Check sheet for the modelled part. Datum: model origin and axes. Units: mm. A direction names the side the tool comes from. Give positions to 0.01 mm unless a question says otherwise; leave off trailing zeros. Order: outer loops, then holes, each group sorted by start corner. A loop starts at its lowest first (then second) coordinate and runs counter-clockwise, first axis right, second up. Notation, with made-up numbers: (-20, -16) -> (13, -16) arc R29 cw to (13, 23) -> close; hole circle Ø3 at (84, -4.5). An arc over 180 degrees is marked (long way). Answer in a Markdown table with one row per item. Add a question column.
(1) Thickness scan on L1, parallel to X at y = 35, z = -40; L2, parallel to Z at x = 26, y = -19.5; L3, parallel to Y at x = -44, z = -14.5. Record the ranges inside material, lowest first. Write a range as [from, to].
(2) Cross-section at C-C (x = 0). Record the cut outline in (y, z).
(3) Go/stop test with flat-tipped pins: pin 1 (5 mm diameter, centred on x = 27.5, y = -14, fed in from -Z); pin 2 (5 mm diameter, centred on y = 11.5, z = 39.5, fed in from +X); pin 3 (1.5 mm diameter, centred on x = 36.5, z = -14, fed in from -Y). Record where each tip stops, or that it passes through.
(4) Release check for a two-part mould opening along Z. For faces 1 (the face through (-60.189, 2.649, 35.827)), 2 (the face through (60.189, 2.717, 35.827)), 3 (the face through (1.08, -4.88, -59.93)), 4 (the face through (0, 0, -65)) record: released by +Z, released by -Z, zero draft, split by the parting line, or undercut.
(5) Cross-section at B-B (y = -3). Record the cut outline in (x, z), then the cut area to 3 significant figures.
(6) Cross-section at D-D (z = -8.5). Record the cut outline in (x, y).
(7) Cross-section at A-A (x = -84). Record the cut outline in (y, z).
(8) Set-up check for faces 5 (the face through (70.99, -22.72, -12.43)), 6 (the face through (-90, 25, -35)), 7 (the face through (90, 25, -35)): record each of +Z, -Z, +X, -X, +Y, -Y from which the full face is reachable in a straight line by a thin tool's end or side.
```python
from build123d import *
from build123d.topology import SkipClean

# Parameters (mm, degrees)
SKETCH1_W                = 180
SKETCH1_H                = 110
BOSS_EXTRUDE1_DEPTH      = 50
BOSS_EXTRUDE2_DEPTH      = 110
CUT_EXTRUDE1_DEPTH       = 146.344418537
BOSS_EXTRUDE5_DEPTH      = 10
BOSS_EXTRUDE5_DEPTH_BACK = 10
SKETCH5_R                = 5


with BuildPart() as part:
    # Sketch1 → Boss-Extrude1 (new body)
    with BuildSketch(Plane(origin=(0, 0, 0), x_dir=(1, 0, 0), z_dir=(0, 1, 0))):
        Rectangle(SKETCH1_W, SKETCH1_H)
    extrude(amount=BOSS_EXTRUDE1_DEPTH)

    # Sketch2 → Boss-Extrude2 (add)
    with BuildSketch(Plane(origin=(-35, 0, -55), x_dir=(1, 0, 0), z_dir=(0, 0, 1))):
        with BuildLine():
            Line((-55, 0), (125, 0))
            ThreePointArc((125, 0), (35, -50), (-55, 0))
        make_face()
    extrude(amount=BOSS_EXTRUDE2_DEPTH)

    # Sketch3 → Cut-Extrude1 (cut, through all)
    with BuildSketch(Plane(origin=(0, 50, 0), x_dir=(1, 0, 0), z_dir=(0, 1, 0))):
        Polygon((-49.118803686, -55), (-90, 15.808309091), (-90, -55), align=None)
    cut_extrude1 = extrude(amount=-CUT_EXTRUDE1_DEPTH, mode=Mode.SUBTRACT)

    # Mirror1: Cut-Extrude1 across plane
    add(cut_extrude1.mirror(Plane(origin=(0, 0, 0), x_dir=(0, 0, 1), z_dir=(1, 0, 0))), mode=Mode.SUBTRACT)

    # Sketch5 → Boss-Extrude5 (add, two sides: drawn at the far end of the back side and taken through both)
    with BuildSketch(Plane(origin=(0, 0, -55), x_dir=(-1, 0, 0), z_dir=(0, 0, -1)).offset(-BOSS_EXTRUDE5_DEPTH_BACK)):
        Circle(SKETCH5_R)
    extrude(amount=BOSS_EXTRUDE5_DEPTH + BOSS_EXTRUDE5_DEPTH_BACK)

    # Sketch4 → Revolve1 (revolve)
    with BuildSketch(Plane(origin=(-60.654801368, 0, 35.019065898), x_dir=(0.49999999999999495, 0, 0.8660254037844417), z_dir=(-0.8660254037844417, 0, 0.49999999999999495))):
        with BuildLine():
            ThreePointArc((-20.965161058, 42.942576489), (4.034838942, 17.942576489), (-20.965161058, -7.057423511))
            Line((-20.965161058, -7.057423511), (-20.965161058, 42.942576489))
        make_face()
    revolve1 = revolve(axis=Axis((-71.137381897, 42.942576489, 16.862703827), (0, -1, 0)))

    # Mirror2: Revolve1 across plane
    add(revolve1.mirror(Plane(origin=(0, 0, 0), x_dir=(0, 0, 1), z_dir=(1, 0, 0))))


with BuildPart() as body_2:
    # Sketch6 → Revolve2 (revolve)
    with SkipClean():  # the faces are left unmerged after this step: merging them gives an invalid solid
        with BuildSketch(Plane.XY):
            with BuildLine():
                ThreePointArc((137.389580355, 89.999956455), (-0.110419645, 227.499956455), (-137.610419645, 89.999956455))
                Line((-137.610419645, 89.999956455), (137.389580355, 89.999956455))
            make_face()
            with BuildLine():
                Line((137.389580355, 89.999956455), (-137.610419645, 89.999956455))
                ThreePointArc((-137.610419645, 89.999956455), (-0.110419645, -47.500043545), (137.389580355, 89.999956455))
            make_face()
        revolve(axis=Axis((-137.610419645, 89.999956455, 0), (1, 0, 0)))
    add(body_2.part.scale(1), mode=Mode.REPLACE)  # the faces are merged on a copy

    # Intersect1: read off the stored shape, not the designer's step
    # Intersect1: intersect part
    add(part.part, mode=Mode.INTERSECT)


solid = body_2.part
```
Answer below:
| question | item | result |
|---|---|---|
| 1 | L1 | x = [-90, 90] |
| 1 | L2 | z = [-55, 55] |
| 1 | L3 | y = [-39.5, 50] |
| 2 | outline | (-36.02, -55) -> (-5, -55) -> (-5, -65) -> (5, -65) -> (5, -55) -> (50, -55) -> (50, 55) -> (-36.02, 55) arc R137.5 ccw to start |
| 3 | pin 1 | stops at z = -55 |
| 3 | pin 2 | stops at x = 84.65 |
| 3 | pin 3 | stops at y = -42.02 |
| 4 | face 1 | undercut |
| 4 | face 2 | undercut |
| 4 | face 3 | zero draft |
| 4 | face 4 | released by -Z |
| 5 | outline | (-88.06, -50.22) arc R101.28 ccw to (-85.15, -55) -> (-4, -55) -> (-4, -65) -> (4, -65) -> (4, -55) -> (84.93, -55) arc R101.28 ccw to (88.06, -49.83) -> (88.06, -12.45) -> (77.96, 5.04) arc R13.65 ccw to (64.31, 28.69) -> (49.12, 55) -> (-49.12, 55) -> (-64.31, 28.69) arc R13.65 ccw to (-77.96, 5.04) -> (-88.06, -12.45) -> close |
| 5 | area | 17,400 mm² |
| 6 | outline | (-85.78, -6.27) arc R106 ccw to (-47.25, -38.89) arc R137.24 ccw to (47.86, -38.58) arc R106 ccw to (85.78, -6.27) -> (85.78, 50) -> (-85.78, 50) -> close |
| 7 | outline | (-8.65, -46.22) arc R108.94 ccw to (-4.04, -55) -> (50, -55) -> (50, -5.42) -> (-8.65, -5.42) -> close; circle Ø42.87 at (17.94, 16.86) |
| 8 | face 5 | +Z, -Z, +X, -Y |
| 8 | face 6 | -Z, -X, +Y, -Y |
| 8 | face 7 | -Z, +X, +Y, -Y |
